Read the model definition and answer for the solid it produces. Units are mm, in the model's axes. Give positions to 0.01 mm unless a question says otherwise; leave off trailing zeros. Order: outer loops, then holes, each group sorted by start corner. A loop starts at its lowest first (then second) coordinate and runs counter-clockwise, first axis right, second up. Notation, with made-up numbers: (-2, 79) -> (34, 79) arc R26 ccw to (34, 109) -> close; hole circle Ø5 at (25, 2.25). An arc over 180 degrees is marked (long way). Use one line per item in the form item = value.
```python
from build123d import *

# Parameters (mm, degrees)
BOSS_EXTRUDE1_DEPTH = 6.35
BOSS_EXTRUDE2_DEPTH = 6.35
CUT_EXTRUDE1_DEPTH  = 176.195383741
SKETCH4_R           = 3
CUT_EXTRUDE2_DEPTH  = 169.439588188
CUT_EXTRUDE3_DEPTH  = 6.35
SKETCH7_R           = 3.81
BOSS_EXTRUDE3_DEPTH = 6.35


with BuildPart() as part:
    # Sketch1 → Boss-Extrude1 (new body)
    with BuildSketch(Plane(origin=(0, 0, 0), x_dir=(0, 0, -1), z_dir=(1, 0, 0))):
        with BuildLine():
            Line((-106.172, 0), (-62.992, 43.18))
            Line((-62.992, 43.18), (0, 43.18))
            Line((0, 43.18), (0, 40.64))
            ThreePointArc((0, 40.64), (-6.479930943, 21.59), (0, 2.54))
            Line((0, 2.54), (0, 0))
            Line((0, 0), (-106.172, 0))
        make_face()
    extrude(amount=BOSS_EXTRUDE1_DEPTH)

    # Sketch2 → Boss-Extrude2 (add)
    with BuildSketch(Plane(origin=(6.35, 0, 0), x_dir=(0, 0, -1), z_dir=(1, 0, 0))):
        Polygon((-68.072, 0), (-169.672, 0), (-144.272, 10.16), (-68.072, 17.78), align=None)
    extrude(amount=-BOSS_EXTRUDE2_DEPTH)

    # Sketch3 → Cut-Extrude1 (cut, through all)
    with BuildSketch(Plane(origin=(6.35, 0, 0), x_dir=(0, 0, -1), z_dir=(1, 0, 0))):
        Polygon((-106.172, 0), (-162.687, 2.794), (-169.672, 0), align=None)
    extrude(amount=-CUT_EXTRUDE1_DEPTH, mode=Mode.SUBTRACT)

    # Sketch4 → Cut-Extrude2 (cut, through all)
    with BuildSketch(Plane(origin=(6.35, 0, 0), x_dir=(0, 0, -1), z_dir=(1, 0, 0))):
        with Locations((-25.4, 31.59)):
            Circle(SKETCH4_R)
        with Locations((-25.4, 11.59)):
            Circle(SKETCH4_R)
        with Locations((-76.2, 11.59)):
            Circle(SKETCH4_R)
    extrude(amount=-CUT_EXTRUDE2_DEPTH, mode=Mode.SUBTRACT)

    # Sketch6 → Cut-Extrude3 (cut)
    with BuildSketch(Plane.ZY):
        Polygon((62.992, 43.18), (90.649777778, 15.522222222), (108.309937594, -2.137937594), (165.318856779, -0.913782118), (157.233600138, 13.290047118), (95.237394621, 20.109839066), align=None)
    extrude(amount=-CUT_EXTRUDE3_DEPTH, mode=Mode.SUBTRACT)

    # Sketch7 → Boss-Extrude3 (add)
    with BuildSketch(Plane.ZY):
        with BuildLine():
            Line((0, 43.18), (-43.481110833, 43.18))
            ThreePointArc((-43.481110833, 43.18), (-53.337069057, 21.59), (-43.481110833, 0))
            Line((-43.481110833, 0), (0, 0))
            Line((0, 0), (0, 2.54))
            ThreePointArc((0, 2.54), (6.479930943, 21.59), (0, 40.64))
            Line((0, 40.64), (0, 43.18))
        make_face()
        with Locations((-24.762069057, 21.59)):
            Circle(SKETCH7_R, mode=Mode.SUBTRACT)
    extrude(amount=-BOSS_EXTRUDE3_DEPTH)


solid = part.part
```
Item 1: The part is cut by section D-D on z = 76.2. Give the vertices of the cut face in (x, y).
Checks:
outline = (0, 0) -> (6.35, 0) -> (6.35, 8.59) -> (0, 8.59) -> close; (0, 14.59) -> (6.35, 14.59) -> (6.35, 29.97) -> (0, 29.97) -> close
Item 2: Straight lines are drawn through the part: L1, parallel to Y at x = 3, z = 25.4; L2, parallel to Y at x = 4.5, z = 27.5; L3, parallel to Z at x = 2.25, y = 32.5. For each, find the intervals that lie inside material, in ascending order. Write a range as from..to.
Checks:
L1 = 0..8.59, 14.59..28.59, 34.59..43.18
L2 = 0..9.45, 13.73..29.45, 33.73..43.18
L3 = -51.17..22.54, 28.26..73.67
Item 3: The part is cut by section A-A on z = 25.4. Give the vertices of the cut face in (x, y).
Checks:
outline = (0, 0) -> (6.35, 0) -> (6.35, 8.59) -> (0, 8.59) -> close; (0, 14.59) -> (6.35, 14.59) -> (6.35, 28.59) -> (0, 28.59) -> close; (0, 34.59) -> (6.35, 34.59) -> (6.35, 43.18) -> (0, 43.18) -> close
Item 4: The part is cut by section C-C on y = 11.59. Give the vertices of the cut face in (x, z).
Checks:
outline = (0, -51.53) -> (6.35, -51.53) -> (6.35, 22.4) -> (0, 22.4) -> close; (0, 28.4) -> (6.35, 28.4) -> (6.35, 73.2) -> (0, 73.2) -> close; (0, 79.2) -> (6.35, 79.2) -> (6.35, 94.58) -> (0, 94.58) -> close
Item 5: Determine the mould class of faces 1 (the cylindrical face through (3.131, 20.131, -21.243)), 2 (the cylindrical face through (3.131, 21.933, -53.335)), 3 (the cylindrical face through (3.22, 32.49, 22.54)), 4 (the flat face through (3, 0, 30)) for opening direction Z: +Z half, -Z half, draft (parallel to the pull), parting line (faces both ways), or undercut.
Checks:
face_1 = undercut
face_2 = -Z half
face_3 = undercut
face_4 = draft
Item 6: Given pin 1 Ø3 at (x, y) = (3.5, 14) entering from -Z; pin 2 Ø5.5 at (y, z) = (11.59, 25.4) entering from -X, each flat-ended and moving along its own axis, determine where each tip first touches the part or whether it passes through.
Checks:
pin_1 = -52.68
pin_2 = through
Item 7: The part is cut by section B-B on x = 3.25. Give the vertices of the cut face in (y, z) (3 decimals), and give its area (3 significant figures).
Checks:
outline = (0, -43.481) arc R28.575 ccw to (43.18, -43.481) -> (43.18, 62.992) -> (0, 106.172) -> close; hole circle Ø6 at (11.59, 25.4); hole circle Ø6 at (11.59, 76.2); hole circle Ø7.62 at (21.59, -24.762); hole circle Ø6 at (31.59, 25.4)
area = 5,690 mm²
